Model file for the job. Use its own axes, mm. A direction names the side the tool comes from. Give positions to 0.01 mm unless a question says otherwise; leave off trailing zeros. Loops run counter-clockwise (first coordinate to the right, second up) from the corner with the lowest first, then second, coordinate; pieces in that order, holes last. Notation, with made-up numbers: (1.25, 62) - (53.25, 62) arc R19 cw to (53.25, 83) - close; hole circle Ø3 at (-1, 10). An arc over 180 degrees is marked (long way). Use a Markdown table: item, result.
from build123d import *

# Parameters (mm, degrees)
ESQUISSE1_R        = 1.5
BOSS_EXTRU_1_DEPTH = 5


with BuildPart() as part:
    # Esquisse1 → Boss.-Extru.1 (new body)
    with BuildSketch(Plane.XY):
        with BuildLine():
            Line((35, 17.5), (35, 0))
            Line((35, 0), (200, 0))
            Line((200, 0), (200, 17.5))
            ThreePointArc((200, 17.5), (205.125631329, 29.874368671), (217.5, 35))
            Line((217.5, 35), (226.881966011, 35))
            ThreePointArc((226.881966011, 35), (227.464766865, 37.401258538), (229.5, 36))
            ThreePointArc((229.5, 36), (229.401258538, 35.464766865), (229.118033989, 35))
            Line((229.118033989, 35), (235, 35))
            Line((235, 35), (235, 65))
            Line((235, 65), (161, 65))
            Line((161, 65), (161, 90))
            Line((161, 90), (74, 90))
            Line((74, 90), (74, 65))
            Line((74, 65), (0, 65))
            Line((0, 65), (0, 35))
            Line((0, 35), (5.881966011, 35))
            ThreePointArc((5.881966011, 35), (6.464766865, 37.401258538), (8.5, 36))
            ThreePointArc((8.5, 36), (8.401258538, 35.464766865), (8.118033989, 35))
            Line((8.118033989, 35), (17.5, 35))
            ThreePointArc((17.5, 35), (29.874368671, 29.874368671), (35, 17.5))
        make_face()
        with Locations((27, 36)):
            Circle(ESQUISSE1_R, mode=Mode.SUBTRACT)
        with Locations((208, 36)):
            Circle(ESQUISSE1_R, mode=Mode.SUBTRACT)
        with Locations((7, 56)):
            Circle(ESQUISSE1_R, mode=Mode.SUBTRACT)
        with Locations((27, 56)):
            Circle(ESQUISSE1_R, mode=Mode.SUBTRACT)
        with Locations((99, 70)):
            Circle(ESQUISSE1_R, mode=Mode.SUBTRACT)
        with Locations((208, 56)):
            Circle(ESQUISSE1_R, mode=Mode.SUBTRACT)
        with Locations((228, 56)):
            Circle(ESQUISSE1_R, mode=Mode.SUBTRACT)
        with Locations((139, 70)):
            Circle(ESQUISSE1_R, mode=Mode.SUBTRACT)
    extrude(amount=BOSS_EXTRU_1_DEPTH)


solid = part.part
(1) Drill centre lines: probe 1 along X at (y, z) = (70, 2.9); probe 2 along Y at (x, z) = (7, 2.45); probe 3 along Y at (x, z) = (99, 1.55). Where is each one in solid material? Low to high. Write a range as [from, to].
Computed:
| item | result |
|---|---|
| probe 1 | [74, 97.5], [100.5, 137.5], [140.5, 161] |
| probe 2 | [37.5, 54.5], [57.5, 65] |
| probe 3 | [0, 68.5], [71.5, 90] |
(2) 3-axis set-ups, long thin cutter, end or side, ignore diameter. For faces 1 (the flat face through (199, 65, 2)), 2 (the flat face through (74, 78, 2)), 3 (the flat face through (3, 35, 2)), 4 (the flat face through (222, 35, 2)), 5 (the flat face through (0, 50, 2)): which of +Z, -Z, +X, -X, +Y, -Y reach the whole face in a straight line?
Computed:
| item | result |
|---|---|
| face 1 | +Z, -Z, +X, +Y |
| face 2 | +Z, -Z, -X, +Y |
| face 3 | +Z, -Z, -X, -Y |
| face 4 | +Z, -Z, +X, -Y |
| face 5 | +Z, -Z, -X, +Y, -Y |
(3) Slice it at C-C, the plane y = 25.5. Write the cut outline in (x, z).
Computed:
| item | result |
|---|---|
| outline | (33.06, 0) - (201.94, 0) - (201.94, 5) - (33.06, 5) - close |
(4) Slice it at B-B, the plane y = 82.5. Write the cut outline in (x, z).
Computed:
| item | result |
|---|---|
| outline | (74, 0) - (161, 0) - (161, 5) - (74, 5) - close |
(5) Pin check, flat tips, straight feed: P1, Ø2.5, axis at x = 222.5, z = 3, coming from the -Y side; P2, Ø1.5, axis at y = 82, z = 3, coming from the -X side; P3, Ø2.5, axis at x = 32.5, z = 3.5, coming from the +Y side. Stop position of each tip, or through.
Computed:
| item | result |
|---|---|
| P1 | y = 35 |
| P2 | x = 74 |
| P3 | y = 65 |
(6) Slice it at A-A, the plane z = 4.15. Count the separate pieces of the cut face and the enclosed holes in it, plus the area to 3 significant figures.
Computed:
| item | result |
|---|---|
| separate pieces | 1 |
| enclosed holes | 8 |
| area | 15,100 mm² |
